Geometry check sheet. Reference: the model listing, model coordinates, mm. Coordinates: 2 decimals unless noted, no trailing zeros. Order: outer loops, then holes, each group sorted by start corner. A loop starts at its lowest first (then second) coordinate and runs counter-clockwise, first axis right, second up. Notation, with made-up numbers: (34, 65) - (76, 65) arc R34 ccw to (76, 102) - close; hole circle Ø4 at (-4, 41.25). An arc over 180 degrees is marked (long way). Put each result on its own line as item: value.
from build123d import *

# Parameters (mm, degrees)
BOSS_EXTRUDE1_DEPTH      = 130
BOSS_EXTRUDE1_DEPTH_BACK = 130
SKETCH3_R                = 10
SKETCH4_R                = 8.5
BOSS_EXTRUDE2_DEPTH      = 2
SKETCH5_R                = 10
BOSS_EXTRUDE3_DEPTH      = 5
BOSS_EXTRUDE4_START      = 2
SKETCH6_R                = 8.5
BOSS_EXTRUDE4_DEPTH      = 2
BOSS_EXTRUDE5_START      = 5
SKETCH7_R                = 10
BOSS_EXTRUDE5_DEPTH      = 5
CUT_EXTRUDE1_DEPTH       = 138.727992797
CUT_EXTRUDE1_DEPTH_BACK  = 138.727992797
SKETCH8_W                = 26
SKETCH8_H                = 2
SKETCH9_R                = 4.5
CUT_EXTRUDE2_DEPTH       = 139.538803249


with BuildPart() as part:
    # Sketch3 → Boss-Extrude1 (new, two sides: drawn at the far end of the back side and taken through both)
    with BuildSketch(Plane.XY.offset(-BOSS_EXTRUDE1_DEPTH_BACK)):
        Circle(SKETCH3_R)
    extrude(amount=BOSS_EXTRUDE1_DEPTH + BOSS_EXTRUDE1_DEPTH_BACK)

    # Sketch4 → Boss-Extrude2 (add)
    with BuildSketch(Plane.XY.offset(130)):
        Circle(SKETCH4_R)
    extrude(amount=BOSS_EXTRUDE2_DEPTH)

    # Sketch5 → Boss-Extrude3 (add)
    with BuildSketch(Plane.XY.offset(132)):
        Circle(SKETCH5_R)
    extrude(amount=BOSS_EXTRUDE3_DEPTH)

    # Sketch6 → Boss-Extrude4 (add)
    with BuildSketch(Plane(origin=(0, 0, -130), x_dir=(-1, 0, 0), z_dir=(0, 0, -1)).offset(BOSS_EXTRUDE4_START)):
        with Locations(Location((0, 0, 0), (0, 0, 180))):
            Circle(SKETCH6_R)
    extrude(amount=-BOSS_EXTRUDE4_DEPTH)

    # Sketch7 → Boss-Extrude5 (add)
    with BuildSketch(Plane(origin=(0, 0, -132), x_dir=(-1, 0, 0), z_dir=(0, 0, -1)).offset(BOSS_EXTRUDE5_START)):
        with Locations(Location((0, 0, 0), (0, 0, 180))):
            Circle(SKETCH7_R)
    extrude(amount=-BOSS_EXTRUDE5_DEPTH)

    # Sketch8 → Cut-Extrude1 (cut, two sides: drawn at the far end of the back side and taken through both)
    with BuildSketch(Plane(origin=(0, 0, 0), x_dir=(0, 0, -1), z_dir=(1, 0, 0)).offset(-CUT_EXTRUDE1_DEPTH_BACK)):
        with Locations((0, 9)):
            Rectangle(SKETCH8_W, SKETCH8_H)
        with Locations((0, -9)):
            Rectangle(SKETCH8_W, SKETCH8_H)
        with BuildLine():
            Line((11, 4), (-11, 4))
            ThreePointArc((-11, 4), (-15, 0), (-11, -4))
            Line((-11, -4), (11, -4))
            ThreePointArc((11, -4), (15, 0), (11, 4))
        make_face()
    extrude(amount=CUT_EXTRUDE1_DEPTH + CUT_EXTRUDE1_DEPTH_BACK, mode=Mode.SUBTRACT)

    # Sketch9 → Cut-Extrude2 (cut, through all)
    with BuildSketch(Plane(origin=(0, 8, 0), x_dir=(1, 0, 0), z_dir=(0, 1, 0))):
        with Locations(Location((0, 0, 0), (0, 0, 270))):
            Circle(SKETCH9_R)
    extrude(amount=-CUT_EXTRUDE2_DEPTH, mode=Mode.SUBTRACT)


solid = part.part
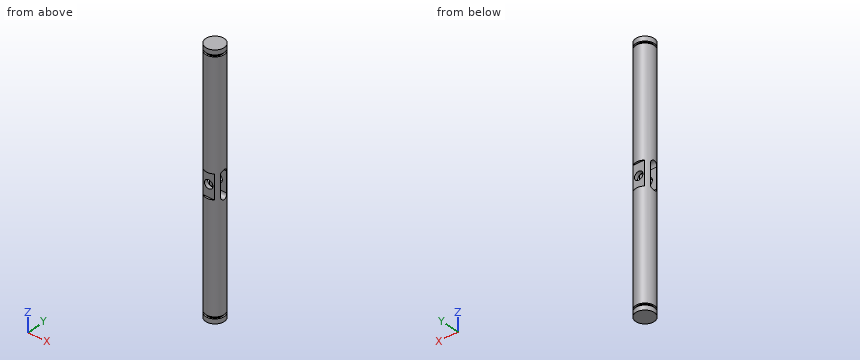
Q1. Section check C-C on z = -103. Record the boundary of the cut face in (x, y), then the cut area to 3 significant figures.
Answer block:
outline: circle Ø20 at (0, 0)
area: 314 mm^2
Q2. Depth check by flat-ended pin: pin 1 Ø1 at (x, z) = (7.5, 40) entering from +Y; pin 2 Ø9 at (x, z) = (0.5, 4.5) entering from +Y; pin 3 Ø2 at (x, z) = (-7, 42) entering from -Y; pin 4 Ø7 at (x, z) = (0, 0) entering from -Y. Enter the tip coordinate at first touch or a pass-through.
Answer block:
pin 1: stops at y = 7.14
pin 2: stops at y = 8
pin 3: stops at y = -8
pin 4: passes through
Q3. Thickness scan on L1, parallel to Z at x = 4, y = 9; L2, parallel to Z at x = 7.25, y = 6.25; L3, parallel to Y at x = 5.25, z = 10. Record the ranges inside material, lowest first. Write a range as [from, to].
Answer block:
L1: z = [-137, -132], [-130, -13], [13, 130], [132, 137]
L2: z = [-137, -132], [-130, 130], [132, 137]
L3: y = [-8, -4], [4, 8]
Q4. Section check B-B on y = 0. Record the boundary of the cut face in (x, z), then the cut area to 3 significant figures.
Answer block:
outline: (-10, -137) - (10, -137) - (10, -132) - (8.5, -132) - (8.5, -130) - (10, -130) - (10, -15) - (-10, -15) - (-10, -130) - (-8.5, -130) - (-8.5, -132) - (-10, -132) - close; (-10, 15) - (10, 15) - (10, 130) - (8.5, 130) - (8.5, 132) - (10, 132) - (10, 137) - (-10, 137) - (-10, 132) - (-8.5, 132) - (-8.5, 130) - (-10, 130) - close
area: 4,870 mm^2
Q5. Section check A-A on z = 0. Record the boundary of the cut face in (x, y), then the cut area to 3 significant figures.
Answer block:
outline: (-9.17, -4) arc R10 ccw to (-6, -8) - (-4.5, -8) - (-4.5, -4) - close; (-9.17, 4) - (-4.5, 4) - (-4.5, 8) - (-6, 8) arc R10 ccw to start; (4.5, -8) - (6, -8) arc R10 ccw to (9.17, -4) - (4.5, -4) - close; (4.5, 4) - (9.17, 4) arc R10 ccw to (6, 8) - (4.5, 8) - close
area: 53.8 mm^2
